from build123d import *

# Parameters (mm, degrees)
F1_DEPTH = 13.97


with BuildPart() as f1:
    # F0 (on Front) → F1 (new body)
    with BuildSketch(Plane.XZ):
        with BuildLine():
            Line((28.575, 9.525), (0, 9.525))
            Line((0, 9.525), (-28.575, 9.525))
            ThreePointArc((-28.575, 9.525), (-43.094035, 10.567071), (-57.15, 14.351))
            Line((-57.15, 14.351), (-123.19, 14.351))
            Line((-123.19, 14.351), (-123.19, -14.351))
            Line((-123.19, -14.351), (-57.15, -14.351))
            ThreePointArc((-57.15, -14.351), (-43.094035, -10.567071), (-28.575, -9.525))
            Line((-28.575, -9.525), (0, -9.525))
            Line((0, -9.525), (28.575, -9.525))
            ThreePointArc((28.575, -9.525), (43.094035, -10.567071), (57.15, -14.351))
            Line((57.15, -14.351), (123.19, -14.351))
            Line((123.19, -14.351), (123.19, 14.351))
            Line((123.19, 14.351), (57.15, 14.351))
            ThreePointArc((57.15, 14.351), (43.094035, 10.567071), (28.575, 9.525))
        make_face()
    extrude(amount=F1_DEPTH)


solid = f1.part
CAD build for the part. Positions are in the model's coordinates, mm. A direction names the side the tool comes from. Coordinates: 2 decimals unless noted, no trailing zeros. Write each loop counter-clockwise with the first axis right and the second up, starting at its lowest first coordinate (ties: lowest second). Pieces come first, ordered by that corner, then holes. Notation, with made-up numbers: M 67.25,-30 L 124.25,-30 A25 cw 124.25,-7 Z; hole C -19,3.5 d6. An arc over 180 degrees is marked long. Return JSON: item names as keys, results as strings.
Item 1: Drop flat-ended pins along their axis: pin 1 Ø1.5 at (x, z) = (20.5, 10.5) entering from +Y; pin 2 Ø2 at (x, y) = (-16.5, -8.5) entering from +Z (3 decimals). Give the stop position or say it passes through.
Findings below:
{"pin 1": "passes through", "pin 2": "stops at z = 9.525"}
Item 2: Two-plate mould, pull along X, no slides. Class faces 4 (the cylindrical face through (42.893, -6.887, -10.533)), 5 (the flat face through (-90, -7, 14.351)), 6 (the flat face through (-123.19, -7, 0)): +X half, -X half, draft (parallel to the pull), parting line (faces both ways), or undercut.
Findings below:
{"face 4": "undercut", "face 5": "draft", "face 6": "-X half"}
Item 3: Slice it at A-A, the plane y = -5. Write the cut outline in (x, z) (3 decimals), and give its area (3 significant figures).
Findings below:
{"outline": "M -123.19,-14.351 L -57.15,-14.351 A76.2 cw -28.575,-9.525 L 28.575,-9.525 A76.2 cw 57.15,-14.351 L 123.19,-14.351 L 123.19,14.351 L 57.15,14.351 A76.2 cw 28.575,9.525 L -28.575,9.525 A76.2 cw -57.15,14.351 L -123.19,14.351 Z", "area": "6,140 mm2"}
Item 4: Slice it at B-B, the plane x = 14.5. Write the cut outline in (y, z) (3 decimals).
Findings below:
{"outline": "M -13.97,-9.525 L 0,-9.525 L 0,9.525 L -13.97,9.525 Z"}
Item 5: Which spindle directions (+Z, -Z, +X, -X, +Y, -Y) get a long thin tool onto all of the face, cutting with end or side? Do faces 1 (the flat face through (0, -7, 9.525)), 2 (the flat face through (0, -7, -9.525)), 3 (the flat face through (90, -7, -14.351)). Say none if no direction does.
Findings below:
{"face 1": "+Z, +Y, -Y", "face 2": "-Z, +Y, -Y", "face 3": "-Z, +X, -X, +Y, -Y"}
Item 6: Probe line 1 (Z direction, x = 29.5, y = -2.5); line 2 (Z direction, x = 55.5, y = -9.75). List the from-to ranges inside material, lowest first. Write a range as from..to.
Findings below:
{"line 1": "z = -9.51..9.51", "line 2": "z = -13.75..13.75"}
